```python
from build123d import *

# Parameters (mm, degrees)
F1_DEPTH = 19.05
F2_R     = 5.08
F3_R     = 5.08


with BuildPart() as f1:
    # F0 (on Front) → F1 (new body)
    with BuildSketch(Plane.XZ):
        with BuildLine():
            Line((135.5546836256, 15.3242284359), (266.7, 50.8))
            Line((266.7, 50.8), (266.7, 127))
            ThreePointArc((266.7, 127), (0, 51.3599310759), (-266.7, 127))
            Line((-266.7, 127), (-266.7, 50.8))
            Line((-266.7, 50.8), (-135.5546836256, 15.3242284359))
            ThreePointArc((-135.5546836256, 15.3242284359), (-123.825, 0), (-135.5546836256, -15.3242284359))
            Line((-135.5546836256, -15.3242284359), (-266.7, -50.8))
            Line((-266.7, -50.8), (-266.7, -127))
            ThreePointArc((-266.7, -127), (0, -51.3599310759), (266.7, -127))
            Line((266.7, -127), (266.7, -50.8))
            Line((266.7, -50.8), (135.5546836256, -15.3242284359))
            ThreePointArc((135.5546836256, -15.3242284359), (123.825, 0), (135.5546836256, 15.3242284359))
        make_face()
    extrude(amount=F1_DEPTH)

    # F2
    f2_edges = [f1.edges().sort_by_distance(p)[0] for p in [
        (0, 0, 51.359931),
        (201.127342, 0, 33.062114),
        (-201.127342, 0, -33.062114),
        (0, 0, -51.359931),
    ]]
    fillet(f2_edges, radius=F2_R)

    # F3
    f3_edges = [f1.edges().sort_by_distance(p)[0] for p in [
        (0, -19.05, 51.359931),
        (-201.127342, -19.05, 33.062114),
        (0, -19.05, -51.359931),
        (201.127342, -5.08, -33.062114),
        (201.127342, -19.05, 33.062114),
    ]]
    fillet(f3_edges, radius=F3_R)


solid = f1.part
```
The model under review builds one solid part; all positions refer to its coordinate system, in mm. A direction names the side the tool comes from. Round coordinates to 2 decimals unless told otherwise and drop trailing zeros. Use a Markdown table: item, result.
Q1. Clearance check with a flat-ended pin moving along its axis: P1, Ø1.5, axis at x = 5, y = -3, coming from the +Z side. State where the tip first meets the part, or that it passes through.
Values:
| item | result |
|---|---|
| P1 | stops at z = 51.21 |
Q2. Tool access review of faces 1 (the cylindrical face through (202.34, -17.52, 34.89)), 2 (the flat face through (202, -9.5, -33.3)), 3 (the flat face through (-200.209, -9.463, -32.814)): name each direction out of +Z, -Z, +X, -X, +Y, -Y from which nothing blocks a thin tool from reaching the whole face with its end or side.
Values:
| item | result |
|---|---|
| face 1 | +X, -Y |
| face 2 | +X, +Y, -Y |
| face 3 | -X, +Y, -Y |
Q3. For line 1 (X direction, y = -5.5, z = -97); line 2 (Z direction, x = 198, y = -18); line 3 (Z direction, x = -186, y = -10.5), list the stretches that pass through material, from the lowest coordinate up.
Values:
| item | result |
|---|---|
| line 1 | x = -266.7 to -210.45, 210.45 to 266.7 |
| line 2 | z = -89.38 to -34.27, 34.27 to 89.38 |
| line 3 | z = -86.64 to -28.97, 28.97 to 86.64 |
Q4. Mouldability with a two-part tool opening along Z and no side actions: class faces 4 (the cylindrical face through (202.34, -1.53, 34.89)), 5 (the flat face through (-266.7, -9, -88)), 6 (the cylindrical face through (-3.931, -9.463, -51.375)) as +Z half, -Z half, draft (parallel to the pull), parting line (faces both ways), or undercut.
Values:
| item | result |
|---|---|
| face 4 | undercut |
| face 5 | draft |
| face 6 | -Z half |
